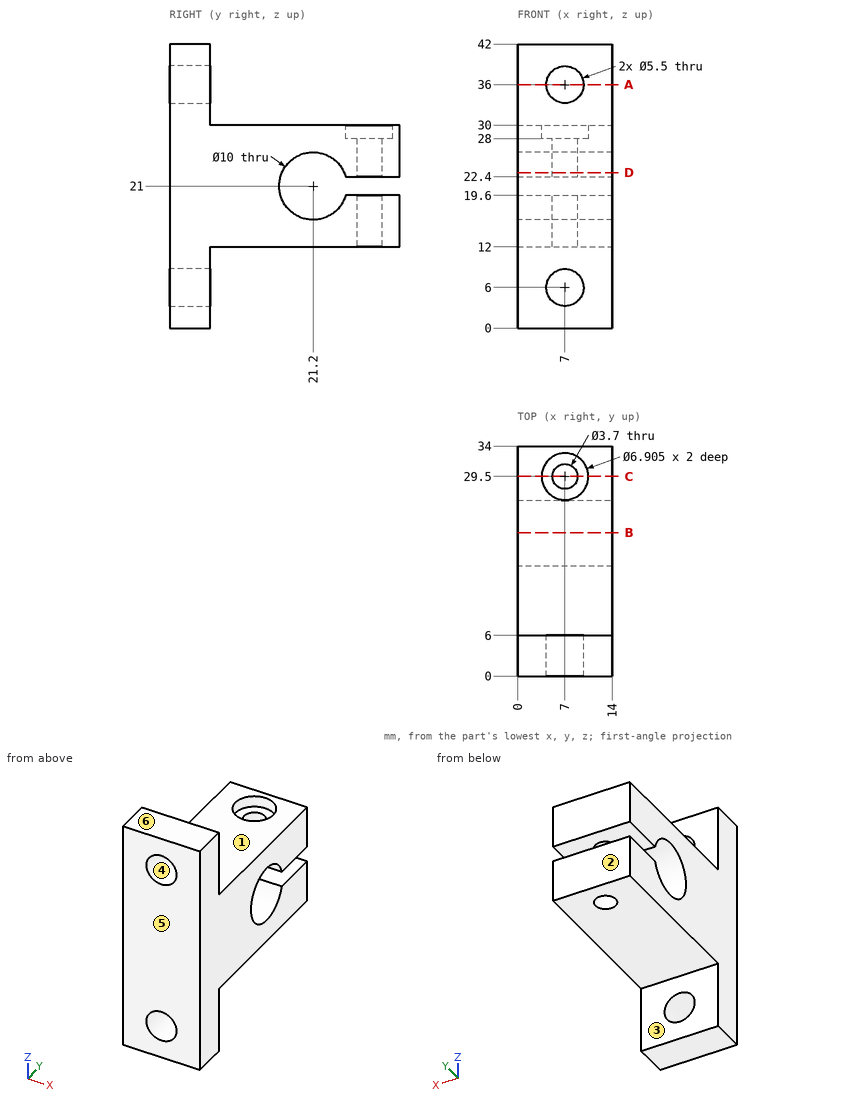
Answer from the drawing. Dimensions are ordinates in mm from the lowest x, y and z of the part. A direction names the side the tool comes from. Round coordinates to 2 decimals unless told otherwise and drop trailing zeros. Order: outer loops, then holes, each group sorted by start corner. A loop starts at its lowest first (then second) coordinate and runs counter-clockwise, first axis right, second up.
1) The part is cut by section B-B on y = 21.2. Write down the section's boundary in (x, z).
2) The mould has two halves that part along Z. Classify the marked faces 4, 5 and 6: released by +Z, released by -Z, zero draft, split by the parting line, or undercut.
3) Straight lines are drawn through the part: L1, parallel to Z at x = 4, y = 32; L2, parallel to X at y = 4, z = 36; L3, parallel to Y at x = 6.5, z = 19.5. For each, find the intervals that lie inside material, in ascending order.
4) The part is cut by section A-A on z = 36. Write down the section's boundary in (x, y).
5) The part is cut by section C-C on y = 29.5. Write down the section's boundary in (x, z).
6) For the marked faces 1, 2 and 3, determine the directions among +Z, -Z, +X, -X, +Y, -Y from which every point of the face is accessible in a straight line to the end or side of a thin tool.
7) The part is cut by section D-D on z = 23. Write down the section's boundary in (x, y), plus the area to 3 significant figures.
8) Flat-ended cylindrical pins translate along their axes: pin 1 (2.5 mm diameter, centred on x = 9.5, y = 31.5, fed in from -Z); pin 2 (7.5 mm diameter, centred on x = 6, y = 30.5, fed in from +Z); pin 3 (13 mm diameter, centred on y = 21.2, z = 21, fed in from -X); pin 4 (2 mm diameter, centred on x = 4, z = 8.5, fed in from +Y). Find the tip coordinate at first contact, or state that the pin passes through.
Resolved:
1. outline: (0, 12) - (14, 12) - (14, 16) - (0, 16) - close; (0, 26) - (14, 26) - (14, 30) - (0, 30) - close
2. face 4: undercut
2. face 5: zero draft
2. face 6: released by +Z
3. L1: z = 12 to 19.6, 22.4 to 30
3. L2: x = 0 to 4.25, 9.75 to 14
3. L3: y = 0 to 16.43, 25.97 to 27.72, 31.28 to 34
4. outline: (0, 0) - (4.25, 0) - (4.25, 6) - (0, 6) - close; (9.75, 0) - (14, 0) - (14, 6) - (9.75, 6) - close
5. outline: (0, 12) - (5.15, 12) - (5.15, 19.6) - (0, 19.6) - close; (0, 22.4) - (5.15, 22.4) - (5.15, 28) - (3.55, 28) - (3.55, 30) - (0, 30) - close; (8.85, 12) - (14, 12) - (14, 19.6) - (8.85, 19.6) - close; (8.85, 22.4) - (14, 22.4) - (14, 30) - (10.45, 30) - (10.45, 28) - (8.85, 28) - close
6. face 1: +Z, +X, -X, +Y
6. face 2: +Z, -Z, +X, -X, +Y
6. face 3: -Z, +X, -X, +Y
7. outline: (0, 0) - (14, 0) - (14, 16.62) - (0, 16.62) - close; (0, 25.78) - (14, 25.78) - (14, 34) - (0, 34) - close; hole circle Ø3.7 at (7, 29.5)
7. area: 337 mm2
8. pin 1: stops at z = 12
8. pin 2: stops at z = 30
8. pin 3: stops at x = 0
8. pin 4: stops at y = 6
